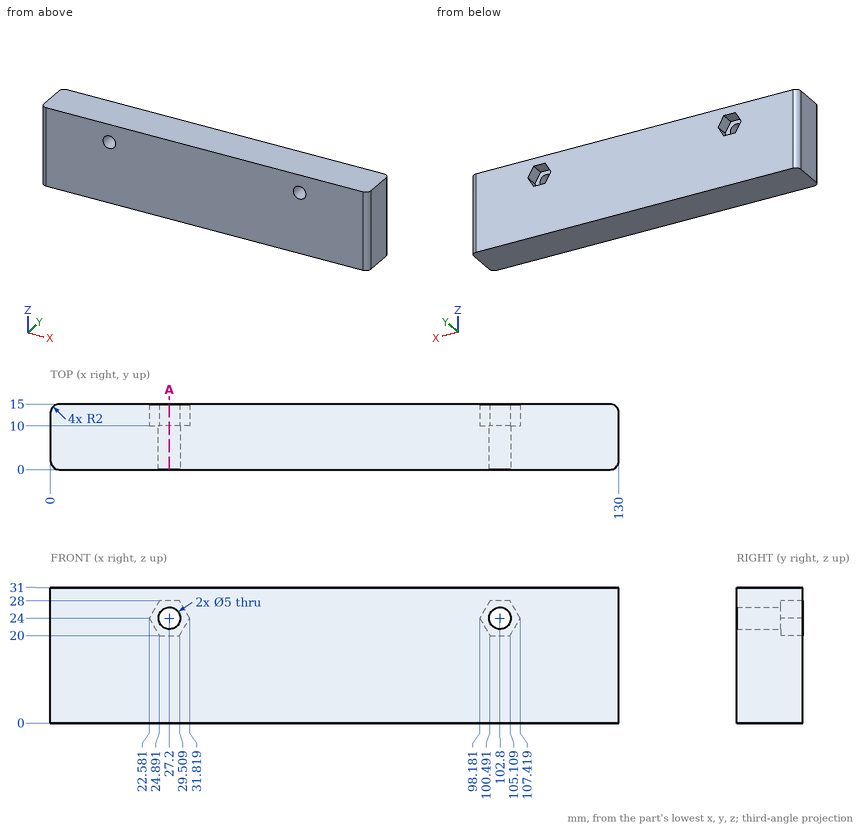
Geometry check sheet. Reference: drawing and pictorial views, mm from the part's lowest x, y, z. Round coordinates to 2 decimals unless told otherwise and drop trailing zeros. Loops run counter-clockwise (first coordinate to the right, second up) from the corner with the lowest first, then second, coordinate; pieces in that order, holes last. Notation, with made-up numbers: (42, -3.75) - (70, -3.75) arc R34 ccw to (70, 30.25) - close; hole circle Ø8 at (-25, 15). An arc over 180 degrees is marked (long way). Answer in a Markdown table with one row per item. Add a question column.
Q1. Section check A-A on x = 27.2. Enter the section's corners in (y, z).
Q2. Gauge pin test, flat ends, axial feed: pin 1 (8 mm diameter, centred on x = 115, z = 8.5, fed in from -Y); pin 2 (2.5 mm diameter, centred on x = 29, z = 25.5, fed in from +Y); pin 3 (4 mm diameter, centred on x = 27.2, z = 24, fed in from -Y). Record the tip position at first contact, or that the pin passes through.
Q3. Material ranges on line 1 (X direction, y = 6, z = 24); line 2 (X direction, y = 7, z = 23); line 3 (Z direction, x = 27.2, y = 4.75), recorded low to high.
Found:
| question | item | result |
|---|---|---|
| 1 | outline | (0, 0) - (15, 0) - (15, 20) - (10, 20) - (10, 21.5) - (0, 21.5) - close; (0, 26.5) - (10, 26.5) - (10, 28) - (15, 28) - (15, 31) - (0, 31) - close |
| 2 | pin 1 | stops at y = 0 |
| 2 | pin 2 | stops at y = 10 |
| 2 | pin 3 | passes through |
| 3 | line 1 | x = 0 to 24.7, 29.7 to 100.3, 105.3 to 130 |
| 3 | line 2 | x = 0 to 24.91, 29.49 to 100.51, 105.09 to 130 |
| 3 | line 3 | z = 0 to 21.5, 26.5 to 31 |
